Model file for the job. Use its own axes, mm. Face numbers are marked on the shaded views. A direction names the side the tool comes from. Coordinates: 2 decimals unless noted, no trailing zeros. Write each loop counter-clockwise with the first axis right and the second up, starting at its lowest first coordinate (ties: lowest second). Pieces come first, ordered by that corner, then holes. Notation, with made-up numbers: M 61.5,27.5 L 114.5,27.5 A30 ccw 114.5,49.5 Z; hole C -24.5,-15 d5. An arc over 180 degrees is marked long. Put each result on its own line as item: value. Start each with the question number.
Q1. Cut at A-A (z = 0). Write the cut outline in (x, y).
Q2. Which spindle directions (+Z, -Z, +X, -X, +Y, -Y) get a long thin tool onto all of the face, cutting with end or side? Do the marked faces 1 and 2. Say none if no direction does.
Q3. Cut at B-B (x = 0). Write the cut outline in (y, z), then the cut area to 3 significant figures.
Q4. Drop flat-ended pins along their axis: pin 1 (1.5 mm diameter, centred on y = 6.5, z = -2, fed in from +X); pin 2 (2 mm diameter, centred on x = -2.5, y = 8.5, fed in from -Z); pin 3 (6 mm diameter, centred on x = 5.5, y = 6, fed in from +Z). Give the stop position or say it passes through.
Q5. Cut at C-C (y = 2.5). Write the cut outline in (x, z).
Q6. Drill centre lines: line 1 along X through (y, z) = (5, 0); line 2 along Y through (x, z) = (-2, -4.5); line 3 along X through (y, z) = (4.5, 1.75). Where is each one in solid material? Low to high.
Q7. Cut at D-D (z = -3.25). Write the cut outline in (x, y), then the cut area to 3 significant figures.
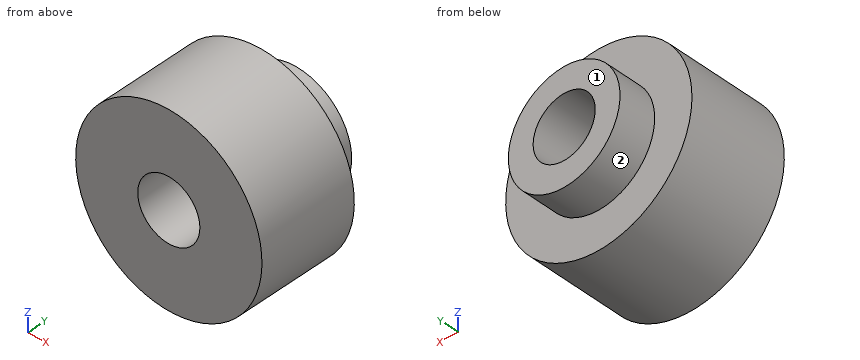
```python
from build123d import *

# Parameters (mm, degrees)
SKETCH1_R           = 7.5
BOSS_EXTRUDE1_DEPTH = 11
SKETCH2_R           = 2.5
CUT_EXTRUDE1_DEPTH  = 16.28070679
CUT_EXTRUDE3_START  = -3
SKETCH3_R           = 7.5
SKETCH3_R_2         = 4.5
CUT_EXTRUDE3_DEPTH  = 3


with BuildPart() as part:
    # Sketch1 → Boss-Extrude1 (new body)
    with BuildSketch(Plane(origin=(0, 0, 0), x_dir=(1, 0, 0), z_dir=(0, 1, 0))):
        with Locations(Location((0, 0, 0), (0, 0, 270))):
            Circle(SKETCH1_R)
    extrude(amount=BOSS_EXTRUDE1_DEPTH)

    # Sketch2 → Cut-Extrude1 (cut, through all)
    with BuildSketch(Plane(origin=(0, 11, 0), x_dir=(1, 0, 0), z_dir=(0, 1, 0))):
        with Locations(Location((0, 0, 0), (0, 0, 270))):
            Circle(SKETCH2_R)
    extrude(amount=-CUT_EXTRUDE1_DEPTH, mode=Mode.SUBTRACT)

    # Sketch3 → Cut-Extrude3 (cut)
    with BuildSketch(Plane(origin=(0, 11, 0), x_dir=(1, 0, 0), z_dir=(0, 1, 0)).offset(CUT_EXTRUDE3_START)):
        with Locations(Location((0, 0, 0), (0, 0, 270))):
            Circle(SKETCH3_R)
        with Locations(Location((0, 0, 0), (0, 0, 270))):
            Circle(SKETCH3_R_2, mode=Mode.SUBTRACT)
    extrude(amount=CUT_EXTRUDE3_DEPTH, mode=Mode.SUBTRACT)


solid = part.part
```
Computed values:
1. outline: M -7.5,0 L -2.5,0 L -2.5,11 L -4.5,11 L -4.5,8 L -7.5,8 Z; M 2.5,0 L 7.5,0 L 7.5,8 L 4.5,8 L 4.5,11 L 2.5,11 Z
2. face 1: +Z, -Z, +X, -X, +Y
2. face 2: +Y
3. outline: M 0,-7.5 L 8,-7.5 L 8,-4.5 L 11,-4.5 L 11,-2.5 L 0,-2.5 Z; M 0,2.5 L 11,2.5 L 11,4.5 L 8,4.5 L 8,7.5 L 0,7.5 Z
3. area: 92.0 mm2
4. pin 1: x = 7.4
4. pin 2: z = -7.32
4. pin 3: z = 7.07
5. outline: C 0,0 d15; hole C 0,0 d5
6. line 1: -7.5 to -2.5, 2.5 to 7.5
6. line 2: 0 to 8
6. line 3: -7.29 to -1.79, 1.79 to 7.29
7. outline: M -6.76,0 L 6.76,0 L 6.76,8 L 3.11,8 L 3.11,11 L -3.11,11 L -3.11,8 L -6.76,8 Z
7. area: 127 mm2
